Verification items for this drawing (mm, ordinates from the low corner). A direction names the side the tool comes from. Coordinates: 2 decimals unless noted, no trailing zeros. Order: outer loops, then holes, each group sorted by start corner. A loop starts at its lowest first (then second) coordinate and runs counter-clockwise, first axis right, second up. Notation, with made-up numbers: M 77,-28 L 124,-28 A15 ccw 124,-22 Z; hole C 59.25,-33.75 d2. An arc over 180 degrees is marked long. Return JSON: item names as keys, results as strings. Group by question number.
1. Set-up check for the marked faces 1 and 2: record each of +Z, -Z, +X, -X, +Y, -Y from which the full face is reachable in a straight line by a thin tool's end or side.
2. Gauge pin test, flat ends, axial feed: pin 1 (8 mm diameter, centred on x = 15.5, z = 7.5, fed in from +Y); pin 2 (1 mm diameter, centred on x = 9, y = 11, fed in from +Z); pin 3 (2 mm diameter, centred on x = 10.5, z = 7.5, fed in from -Y); pin 4 (10 mm diameter, centred on x = 9.5, y = 7, fed in from +Z). Record the tip position at first contact, or that the pin passes through.
3. Section check A-A, the plane x = 10. Record the cut outline in (y, z), plus the area to 3 significant figures.
4. Section check C-C, the plane z = 12.75. Record the cut outline in (x, y), plus the area to 3 significant figures.
5. Material ranges on line 1 along Y through (x, z) = (10, 13); line 2 along X through (y, z) = (8, 11.5); line 3 along Z through (x, y) = (16, 9.75), recorded low to high.
6. Mould release check, pull along Y, two halves, no side actions. Record for the marked faces 3, 4 and 5: +Y half, -Y half, draft (parallel to the pull), parting line (faces both ways), or undercut.
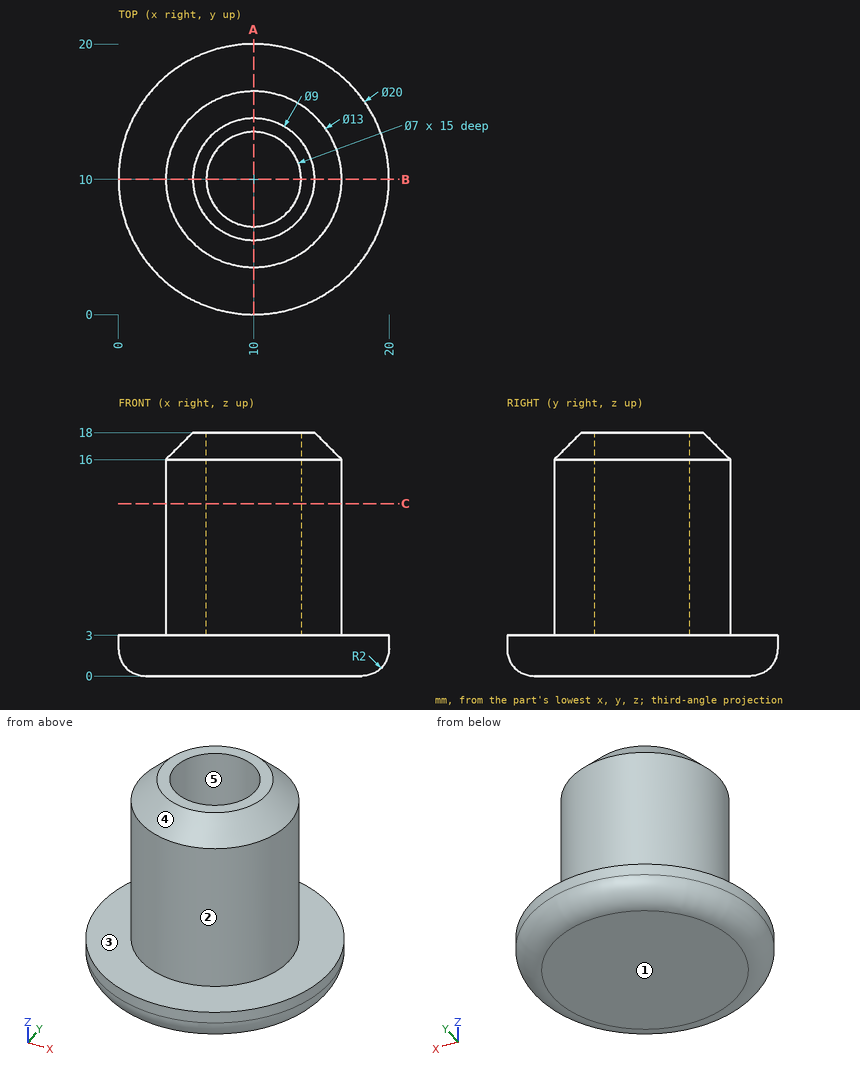
Answers follow:
{
 "1": {"face 1": "-Z, +X, -X, +Y, -Y", "face 2": "+Z"},
 "2": {"pin 1": "y = 16.32", "pin 2": "z = 3", "pin 3": "y = 3.5", "pin 4": "z = 18"},
 "3": {"outline": "M 0,2 A2 ccw 2,0 L 18,0 A2 ccw 20,2 L 20,3 L 16.5,3 L 16.5,16 L 14.5,18 L 13.5,18 L 13.5,3 L 6.5,3 L 6.5,18 L 5.5,18 L 3.5,16 L 3.5,3 L 0,3 Z", "area": "144 mm^2"},
 "4": {"outline": "C 10,10 d13; hole C 10,10 d7", "area": "94.2 mm^2"},
 "5": {"line 1": "3.5 to 6.5, 13.5 to 16.5", "line 2": "3.82 to 7.13, 12.87 to 16.18", "line 3": "0 to 16.49"},
 "6": {"face 3": "draft", "face 4": "parting line", "face 5": "undercut"}
}
